from build123d import *

# Parameters (mm, degrees)
SKETCH1_R           = 10
SKETCH1_R_2         = 1
BOSS_EXTRUDE1_DEPTH = 3
SKETCH2_R           = 2
CUT_EXTRUDE1_DEPTH  = 1
SKETCH4_R           = 1.5
BOSS_EXTRUDE2_DEPTH = 3


with BuildPart() as part:
    # Sketch1 → Boss-Extrude1 (new body)
    with BuildSketch(Plane(origin=(0, 0, 0), x_dir=(1, 0, 0), z_dir=(0, 1, 0))):
        with Locations(Location((0, 0, 0), (0, 0, 270))):
            Circle(SKETCH1_R)
        with Locations(Location((0, 5.773502692, 0), (0, 0, 270))):
            Circle(SKETCH1_R_2, mode=Mode.SUBTRACT)
        with Locations(Location((-5, -2.886751346, 0), (0, 0, 270))):
            Circle(SKETCH1_R_2, mode=Mode.SUBTRACT)
        with Locations(Location((5, -2.886751346, 0), (0, 0, 270))):
            Circle(SKETCH1_R_2, mode=Mode.SUBTRACT)
    extrude(amount=BOSS_EXTRUDE1_DEPTH)

    # Sketch2 → Cut-Extrude1 (cut)
    with BuildSketch(Plane(origin=(0, 3, 0), x_dir=(1, 0, 0), z_dir=(0, 1, 0))):
        with Locations(Location((0, 5.773502692, 0), (0, 0, 270))):
            Circle(SKETCH2_R)
        with Locations(Location((-5, -2.886751346, 0), (0, 0, 270))):
            Circle(SKETCH2_R)
        with Locations(Location((5, -2.886751346, 0), (0, 0, 270))):
            Circle(SKETCH2_R)
    extrude(amount=-CUT_EXTRUDE1_DEPTH, mode=Mode.SUBTRACT)

    # Sketch4 → Boss-Extrude2 (add)
    with BuildSketch(Plane(origin=(0, 3, 0), x_dir=(1, 0, 0), z_dir=(0, 1, 0))):
        with Locations(Location((0, 0, 0), (0, 0, 270))):
            Circle(SKETCH4_R)
    extrude(amount=BOSS_EXTRUDE2_DEPTH)


solid = part.part
The listing builds one solid part. Answer for the finished solid, in the listing's coordinates (mm). A direction names the side the tool comes from. Coordinates: 2 decimals unless noted, no trailing zeros. Order: outer loops, then holes, each group sorted by start corner. A loop starts at its lowest first (then second) coordinate and runs counter-clockwise, first axis right, second up.
Q1. A cutting plane is placed at C-C, the plane z = 0. Write down the section's boundary in (x, y).
Q2. Which of the six approach directions +Z, -Z, +X, -X, +Y, -Y give full straight-line access (tool end or side, diameter ignored) to faces 1 (the face through (6, 2, 2)), 2 (the face through (-0.38, 0.99, -4.85))?
Q3. For a pull along X with two mould halves and no side action, classify faces 3 (the face through (0, 0, 0)), 4 (the face through (5.843, 0.986, 3.424)), 5 (the face through (-9.76, 1.48, -2.17)) as pulls with the +X half, pulls with the -X half, needs draft (parallel to the pull), parting line crosses it, or undercut.
Q4. A cutting plane is placed at D-D, the plane y = 2.5. Write down the section's boundary in (x, z).
Q5. Consider line 1 (Z direction, x = -3.25, y = 2.6) (1 decimal); line 2 (Y direction, x = -0.25, z = -8.25); line 3 (Z direction, x = 6.5, y = 2.5). Determine where each line is inside the solid, lowest interval first.
Q6. Given P1, Ø2, axis at x = 6, z = 2.5, coming from the +Y side; P2, Ø2.5, axis at x = -5, z = 2.89, coming from the +Y side, each flat-ended and moving along its own axis, determine where each tip first touches the part or whether it passes through.
Q7. A cutting plane is placed at B-B, the plane z = -5.25. Write down the section's boundary in (x, y).
Q8. A cutting plane is placed at A-A, the plane x = 0. Write down the section's boundary in (y, z), and give its area (3 significant figures).
Answers follow:
1. outline: (-10, 0) - (10, 0) - (10, 3) - (1.5, 3) - (1.5, 6) - (-1.5, 6) - (-1.5, 3) - (-10, 3) - close
2. face 1: +Y
2. face 2: +Y, -Y
3. face 3: needs draft
3. face 4: undercut
3. face 5: parting line crosses it
4. outline: circle Ø20 at (0, 0); hole circle Ø4 at (-5, 2.89); hole circle Ø4 at (0, -5.77); hole circle Ø4 at (5, 2.89)
5. line 1: z = -9.5 to 1.9, 3.9 to 9.5
5. line 2: y = 0 to 3
5. line 3: z = -7.6 to 1.56, 4.21 to 7.6
6. P1: stops at y = 3
6. P2: stops at y = 2
7. outline: (-8.51, 0) - (-0.85, 0) - (-0.85, 2) - (-1.93, 2) - (-1.93, 3) - (-8.51, 3) - close; (0.85, 0) - (8.51, 0) - (8.51, 3) - (1.93, 3) - (1.93, 2) - (0.85, 2) - close
8. outline: (0, -10) - (3, -10) - (3, -7.77) - (2, -7.77) - (2, -6.77) - (0, -6.77) - close; (0, -4.77) - (2, -4.77) - (2, -3.77) - (3, -3.77) - (3, -1.5) - (6, -1.5) - (6, 1.5) - (3, 1.5) - (3, 10) - (0, 10) - close
8. area: 61.0 mm2
